Input: part model. Units: mm. Frame: model coordinates. Give positions to 0.01 mm unless a question says otherwise; leave off trailing zeros. Write each loop counter-clockwise with the first axis right and the second up, starting at its lowest first coordinate (ties: lowest second). Pieces come first, ordered by that corner, then holes.
```python
from build123d import *

# Parameters (mm, degrees)
CROQUIS3_W              = 700
CROQUIS3_H              = 300
CROQUIS3_H_2            = 30
CROQUIS3_W_2            = 30
CROQUIS3_H_3            = 50
SALIENTE_EXTRUIR1_DEPTH = 10
CROQUIS5_R              = 5
CORTAR_EXTRUIR1_DEPTH   = 10
MATRIZL1_COUNT          = 16
MATRIZL1_PITCH          = 40
MATRIZL1_COUNT_DIR2     = 7
MATRIZL1_PITCH_DIR2     = 40
CROQUIS6_R              = 5
CORTAR_EXTRUIR2_DEPTH   = 10


with BuildPart() as part:
    # Croquis3 → Saliente-Extruir1 (new body)
    with BuildSketch(Plane(origin=(0, 0, 0), x_dir=(1, 0, 0), z_dir=(0, 1, 0))):
        Rectangle(CROQUIS3_W, CROQUIS3_H)
        with Locations((0, -165)):
            Rectangle(CROQUIS3_W, CROQUIS3_H_2)
        with Locations((365, 20)):
            Rectangle(CROQUIS3_W_2, CROQUIS3_H_3)
        with Locations((-365, 20)):
            Rectangle(CROQUIS3_W_2, CROQUIS3_H_3)
    extrude(amount=SALIENTE_EXTRUIR1_DEPTH)

    # Croquis5 → Cortar-Extruir1 (cut)
    with BuildSketch(Plane(origin=(0, 10, 0), x_dir=(1, 0, 0), z_dir=(0, 1, 0))):
        with Locations(Location((-310, 110, 0), (0, 0, 270))):
            Circle(CROQUIS5_R)
    cortar_extruir1 = extrude(amount=-CORTAR_EXTRUIR1_DEPTH, mode=Mode.SUBTRACT)

    # MatrizL1: Cortar-Extruir1 16 × 7
    with Locations(*[(i * MATRIZL1_PITCH, 0, j * MATRIZL1_PITCH_DIR2) for i in range(MATRIZL1_COUNT) for j in range(MATRIZL1_COUNT_DIR2) if (i, j) != (0, 0)]):
        add(cortar_extruir1, mode=Mode.SUBTRACT)

    # Croquis6 → Cortar-Extruir2 (cut)
    with BuildSketch(Plane(origin=(0, 10, 0), x_dir=(1, 0, 0), z_dir=(0, 1, 0))):
        with Locations(Location((-365, 20, 0), (0, 0, 270))):
            Circle(CROQUIS6_R)
        with Locations(Location((365, 20, 0), (0, 0, 270))):
            Circle(CROQUIS6_R)
    extrude(amount=-CORTAR_EXTRUIR2_DEPTH, mode=Mode.SUBTRACT)


solid = part.part
```
Item 1: Ray query, line 1 (X direction, y = 3.25, z = -19); line 2 (X direction, y = 1, z = 145). Return the intervals inside material, ascending.
Item 2: Section A-A (y = 8). Give the number of separate pieces and of enclosed holes in the cut face, and give its area (3 significant figures).
Item 3: Pin query (flat end, axial travel): pin 1 (8 mm diameter, centred on x = -110, z = 130, fed in from -Y); pin 2 (3 mm diameter, centred on x = 215, z = 91.5, fed in from -Y); pin 3 (5 mm diameter, centred on x = 365, y = 5, fed in from -Z); pin 4 (5 mm diameter, centred on y = 6, z = -91.5, fed in from +X). Return the tip coordinate at first contact, or that it passes through.
Item 4: Section B-B (z = 110). Return loops of the section in (x, y), and give its area (3 significant figures).
Solved:
1. line 1: x = -380 to -369.9, -360.1 to 360.1, 369.9 to 380
1. line 2: x = -350 to 350
2. separate pieces: 1
2. enclosed holes: 114
2. area: 225,000 mm2
3. pin 1: passes through
3. pin 2: stops at y = 0
3. pin 3: stops at z = -45
3. pin 4: stops at x = 350
4. outline: (-350, 0) - (350, 0) - (350, 10) - (-350, 10) - close
4. area: 7,000 mm2
